Geometry check sheet. Reference: drawing and pictorial views, mm from the part's lowest x, y, z. A direction names the side the tool comes from. Coordinates: 2 decimals unless noted, no trailing zeros. Write each loop counter-clockwise with the first axis right and the second up, starting at its lowest first coordinate (ties: lowest second). Pieces come first, ordered by that corner, then holes. Notation, with made-up numbers: M 15,56 L 55,56 A14 cw 55,75 Z; hole C 42.25,52.5 d5. An arc over 180 degrees is marked long. One line per item, written item: value.
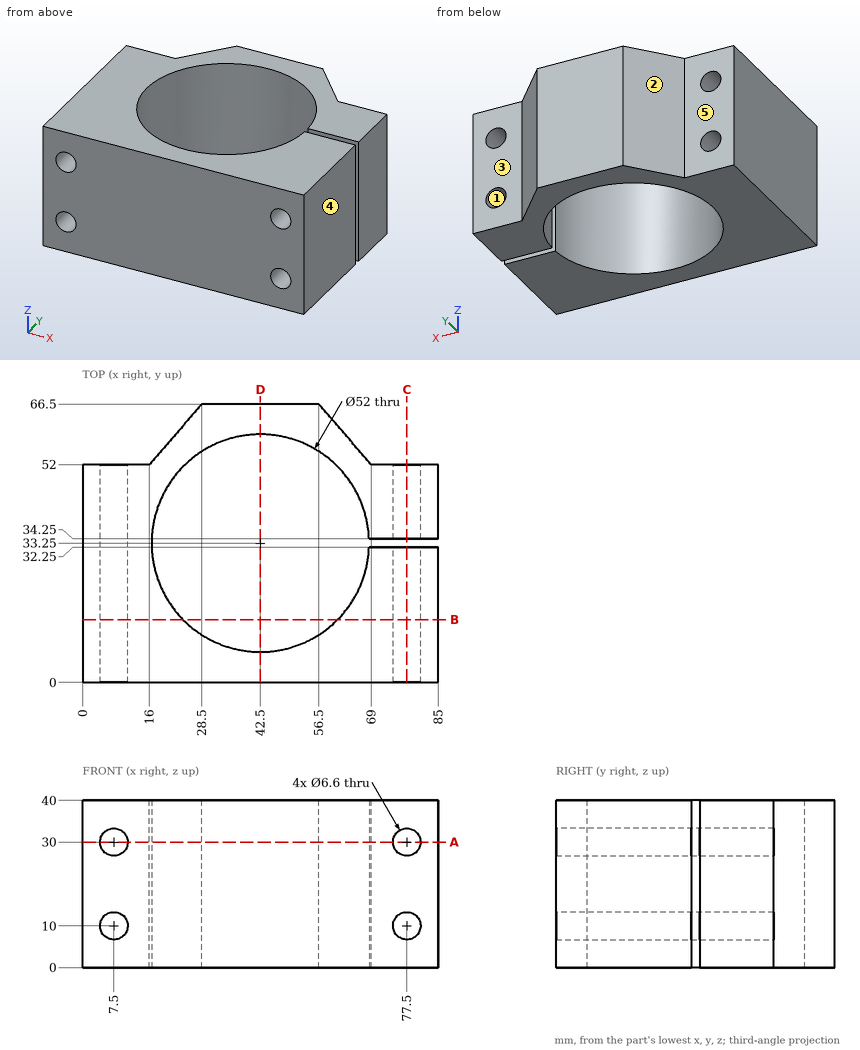
Item 1: Access from +Z, -Z, +X, -X, +Y, -Y to the whole of each face (thin tool, end or side, straight path). Record for the marked faces 4 and 5.
The answers:
face 4: +Z, -Z, +X, +Y, -Y
face 5: +Z, -Z, -X, +Y
Item 2: Cross-section at D-D, the plane x = 42.5. Enter the section's corners in (y, z), and give its area (3 significant figures).
The answers:
outline: M 0,0 L 7.25,0 L 7.25,40 L 0,40 Z; M 59.25,0 L 66.5,0 L 66.5,40 L 59.25,40 Z
area: 580 mm²
Item 3: Cross-section at A-A, the plane z = 30. Enter the section's corners in (x, y), and give its area (3 significant figures).
The answers:
outline: M 0,0 L 4.2,0 L 4.2,52 L 0,52 Z; M 10.8,0 L 74.2,0 L 74.2,32.25 L 68.48,32.25 A26 cw long 68.48,34.25 L 74.2,34.25 L 74.2,52 L 69,52 L 56.5,66.5 L 28.5,66.5 L 16,52 L 10.8,52 Z; M 80.8,0 L 85,0 L 85,32.25 L 80.8,32.25 Z; M 80.8,34.25 L 85,34.25 L 85,52 L 80.8,52 Z
area: 2,180 mm²
Item 4: Draft check along X on the marked faces 1, 2 and 3. Enter one of: released by +X, released by -X, zero draft, split by the parting line, or undercut.
The answers:
face 1: undercut
face 2: released by -X
face 3: zero draft
Item 5: Cross-section at C-C, the plane x = 77.5. Enter the section's corners in (y, z).
The answers:
outline: M 0,0 L 32.25,0 L 32.25,6.7 L 0,6.7 Z; M 0,13.3 L 32.25,13.3 L 32.25,26.7 L 0,26.7 Z; M 0,33.3 L 32.25,33.3 L 32.25,40 L 0,40 Z; M 34.25,0 L 52,0 L 52,6.7 L 34.25,6.7 Z; M 34.25,13.3 L 52,13.3 L 52,26.7 L 34.25,26.7 Z; M 34.25,33.3 L 52,33.3 L 52,40 L 34.25,40 Z
Item 6: Go/stop test with flat-tipped pins: P1, Ø8, axis at x = 70.5, z = 22.5, coming from the -Y side; P2, Ø17.5, axis at x = 8.5, z = 21, coming from the +Y side; P3, Ø13, axis at x = 74.5, z = 23.5, coming from the +Y side; P4, Ø5, axis at x = 75, z = 22.5, coming from the +Y side. Record where each tip stops, or that it passes through.
The answers:
P1: stops at y = 0
P2: stops at y = 53.45
P3: stops at y = 53.16
P4: stops at y = 52
Item 7: Cross-section at B-B, the plane y = 15. Enter the section's corners in (x, z).
The answers:
outline: M 0,0 L 23.98,0 L 23.98,40 L 0,40 Z; M 61.02,0 L 85,0 L 85,40 L 61.02,40 Z; hole C 7.5,10 d6.6; hole C 7.5,30 d6.6; hole C 77.5,10 d6.6; hole C 77.5,30 d6.6
Item 8: Scan lines: line 1 (X direction, y = 7, z = 10); line 2 (Y direction, x = 75, z = 12.5); line 3 (X direction, y = 39, z = 10). Record each from-to range of solid material in increasing order.
The answers:
line 1: x = 0 to 4.2, 10.8 to 74.2, 80.8 to 85
line 2: y = 0 to 32.25, 34.25 to 52
line 3: x = 0 to 4.2, 10.8 to 17.14, 67.86 to 74.2, 80.8 to 85
